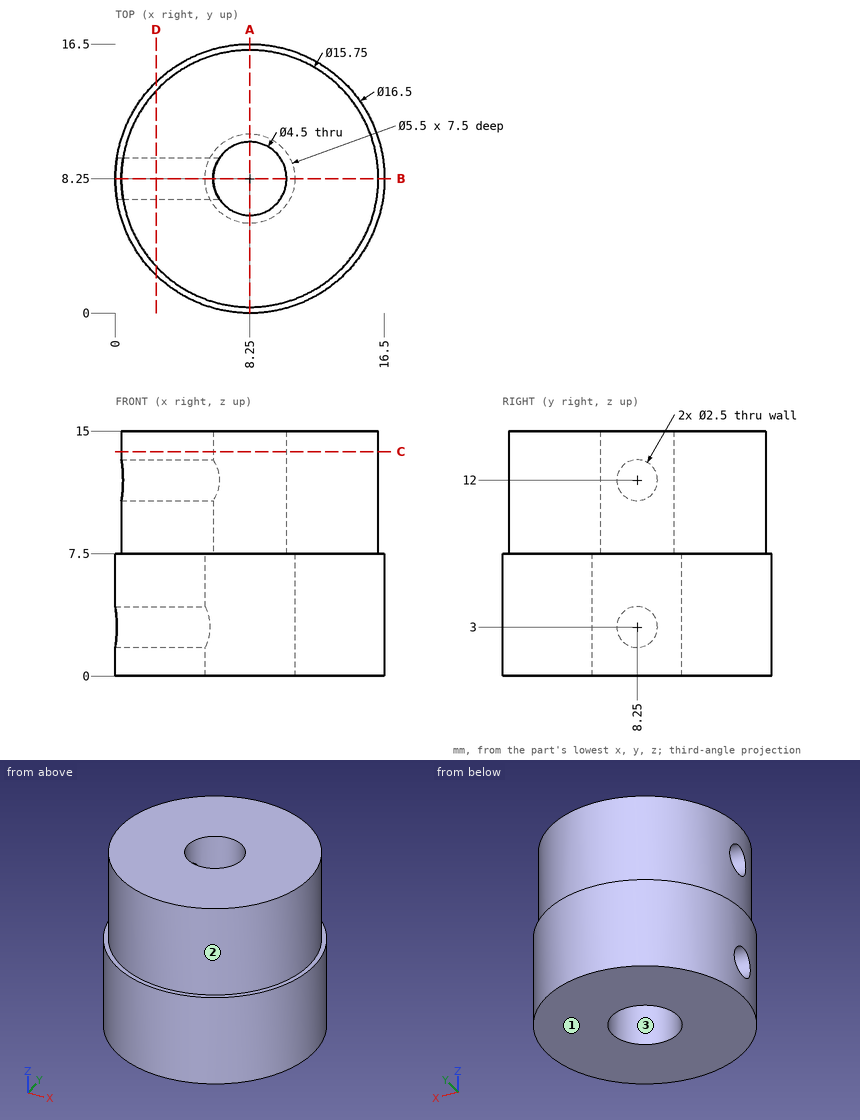
Verification items for this drawing (mm, ordinates from the low corner). Give positions to 0.01 mm unless a question says otherwise; leave off trailing zeros. Loops run counter-clockwise (first coordinate to the right, second up) from the corner with the lowest first, then second, coordinate; pieces in that order, holes last. Notation, with made-up numbers: (77, 0.5) - (84, 0.5) arc R31 ccw to (84, 33.5) - close; hole circle Ø10 at (16, 14.5). An arc over 180 degrees is marked (long way). Write item = value, one per line. Start each with the question number.
Q1. Cross-section at A-A, the plane x = 8.25. Enter the section's corners in (y, z) (3 decimals).
Q2. Cross-section at C-C, the plane z = 13.75. Enter the section's corners in (x, y) (3 decimals).
Q3. Cross-section at D-D, the plane x = 2.5. Enter the section's corners in (y, z), and give its area (3 significant figures).
Q4. Depth check by flat-ended pin: P1, Ø8, axis at x = 13.5, z = 6, coming from the -Y side; P2, Ø5, axis at x = 13, z = 5, coming from the -Y side; P3, Ø4, axis at y = 2.5, z = 9, coming from the +X side. Enter the tip coordinate at first touch or a pass-through.
Q5. Thickness scan on line 1 (Y direction, x = 8.25, z = 11.5) (3 decimals); line 2 (Y direction, x = 2.5, z = 11.5); line 3 (Z direction, x = 1.5, y = 7.5). Record the ranges inside material, lowest first.
Q6. Mould release check, pull along Y, two halves, no side actions. Record for the marked faces 1, 2 and 3: released by +Y, released by -Y, zero draft, split by the parting line, or undercut.
Q7. Cross-section at B-B, the plane y = 8.25. Enter the section's corners in (x, z) (3 decimals), and give its area (3 significant figures).
Answer key:
q1.outline = (0, 0) - (5.5, 0) - (5.5, 7.5) - (6, 7.5) - (6, 15) - (0.375, 15) - (0.375, 7.5) - (0, 7.5) - close; (10.5, 7.5) - (11, 7.5) - (11, 0) - (16.5, 0) - (16.5, 7.5) - (16.125, 7.5) - (16.125, 15) - (10.5, 15) - close
q2.outline = circle Ø15.75 at (8.25, 8.25); hole circle Ø4.5 at (8.25, 8.25)
q3.outline = (2.33, 0) - (14.17, 0) - (14.17, 7.5) - (13.63, 7.5) - (13.63, 15) - (2.87, 15) - (2.87, 7.5) - (2.33, 7.5) - close; hole circle Ø2.5 at (8.25, 3); hole circle Ø2.5 at (8.25, 12)
q3.area = 160 mm^2
q4.P1 = 0.1
q4.P2 = 0.31
q4.P3 = 15.21
q5.line_1 = 0.375 to 6, 10.5 to 16.125
q5.line_2 = 2.87 to 7.1, 9.4 to 13.63
q5.line_3 = 0 to 2, 4 to 11, 13 to 15
q6.face_1 = zero draft
q6.face_2 = split by the parting line
q6.face_3 = undercut
q7.outline = (0, 0) - (5.5, 0) - (5.5, 1.75) - (0, 1.75) - close; (0, 4.25) - (5.5, 4.25) - (5.5, 7.5) - (6, 7.5) - (6, 10.75) - (0.375, 10.75) - (0.375, 7.5) - (0, 7.5) - close; (0.375, 13.25) - (6, 13.25) - (6, 15) - (0.375, 15) - close; (10.5, 7.5) - (11, 7.5) - (11, 0) - (16.5, 0) - (16.5, 7.5) - (16.125, 7.5) - (16.125, 15) - (10.5, 15) - close
q7.area = 139 mm^2
